from build123d import *

# Parameters (mm, degrees)
F1_DEPTH = 3


with BuildPart() as f1:
    # F0 (on Front) → F1 (new body)
    with BuildSketch(Plane.XZ):
        Polygon((-52.314732, 2.8), (-52.314732, 0), (-52.314732, -2.8), (-55.314732, -2.8), (-55.314732, -12.8), (-52.314732, -12.8), (-52.314732, -19.8), (-35.314732, -19.8), (-35.314732, -22.8), (-25.314732, -22.8), (-25.314732, -19.8), (-16.314732, -19.8), (-16.314732, -13.3), (-17.314732, -13.3), (-17.314732, -11.3), (-16.314732, -11.3), (-16.314732, -7.8), (-14.314732, -7.8), (-14.314732, -11.3), (-13.314732, -11.3), (-13.314732, -13.3), (-14.314732, -13.3), (-14.314732, -19.8), (-5.314732, -19.8), (-5.314732, -22.8), (-0.314732, -22.8), (4.685268, -22.8), (4.685268, -19.8), (13.685268, -19.8), (13.685268, -13.3), (12.685268, -13.3), (12.685268, -11.3), (13.685268, -11.3), (13.685268, -7.8), (15.685268, -7.8), (15.685268, -11.3), (16.685268, -11.3), (16.685268, -13.3), (15.685268, -13.3), (15.685268, -19.8), (24.685268, -19.8), (24.685268, -22.8), (34.685268, -22.8), (34.685268, -19.8), (51.685268, -19.8), (51.685268, -12.8), (54.685268, -12.8), (54.685268, -2.8), (51.685268, -2.8), (51.685268, 0), (51.685268, 2.8), (54.685268, 2.8), (54.685268, 12.8), (51.685268, 12.8), (51.685268, 19.8), (34.685268, 19.8), (34.685268, 22.8), (24.685268, 22.8), (24.685268, 19.8), (15.685268, 19.8), (15.685268, 13.3), (16.685268, 13.3), (16.685268, 11.3), (15.685268, 11.3), (15.685268, 7.8), (13.685268, 7.8), (13.685268, 11.3), (12.685268, 11.3), (12.685268, 13.3), (13.685268, 13.3), (13.685268, 19.8), (4.685268, 19.8), (4.685268, 22.8), (-0.314732, 22.8), (-5.314732, 22.8), (-5.314732, 19.8), (-14.314732, 19.8), (-14.314732, 13.3), (-13.314732, 13.3), (-13.314732, 11.3), (-14.314732, 11.3), (-14.314732, 7.8), (-16.314732, 7.8), (-16.314732, 11.3), (-17.314732, 11.3), (-17.314732, 13.3), (-16.314732, 13.3), (-16.314732, 19.8), (-25.314732, 19.8), (-25.314732, 22.8), (-35.314732, 22.8), (-35.314732, 19.8), (-52.314732, 19.8), (-52.314732, 12.8), (-55.314732, 12.8), (-55.314732, 2.8), align=None)
    extrude(amount=F1_DEPTH)


solid = f1.part
The listing builds one solid part. Answer for the finished solid, in the listing's coordinates (mm). A direction names the side the tool comes from. Coordinates: 2 decimals unless noted, no trailing zeros. Write each loop counter-clockwise with the first axis right and the second up, starting at its lowest first coordinate (ties: lowest second). Pieces come first, ordered by that corner, then holes. Notation, with made-up numbers: (-13, 76.5) - (21, 76.5) arc R11 ccw to (21, 83.5) - close; hole circle Ø3 at (28, 3). An arc over 180 degrees is marked (long way). Answer as CSV lines item,"result".
1. Find section A-A (z = -15.5). Give the vertices of the cut face in (x, y), plus the area to 3 significant figures.
Computed values:
outline,"(-52.31, -3) - (-16.31, -3) - (-16.31, 0) - (-52.31, 0) - close; (-14.31, -3) - (13.69, -3) - (13.69, 0) - (-14.31, 0) - close; (15.69, -3) - (51.69, -3) - (51.69, 0) - (15.69, 0) - close"
area,"300 mm²"
2. Determine the mould class of faces 4 (the flat face through (-44, -1, -19.8)), 5 (the flat face through (16.685, -1, -12)), 6 (the flat face through (15.685, -1, 17)), 7 (the flat face through (51.685, -1, -16)) for opening direction X: +X half, -X half, draft (parallel to the pull), parting line (faces both ways), or undercut.
Computed values:
face 4,"draft"
face 5,"undercut"
face 6,"undercut"
face 7,"+X half"
3. A tool of negligible diameter and unlimited length cuts with its end or side. For faces 1 (the flat face through (-13.315, -1, -12)), 2 (the flat face through (20, -1, 19.8)), 3 (the flat face through (-21, -1, -19.8)), from which of +Z, -Z, +X, -X, +Y, -Y can it reach the whole face along a straight path? Write none if from no direction.
Computed values:
face 1,"+Y, -Y"
face 2,"+Z, +Y, -Y"
face 3,"-Z, +Y, -Y"
4. Given P1, Ø1.1, axis at x = 13.5, y = -1, coming from the +Z side; P2, Ø10, axis at x = 37.5, z = -8.5, coming from the +Y side; P3, Ø1.1, axis at x = -13.5, y = -1, coming from the -Z side; P4, Ø1, axis at y = -2, z = -2, coming from the +X side, each flat-ended and moving along its own axis, determine where each tip first touches the part or whether it passes through.
Computed values:
P1,"stops at z = 19.8"
P2,"stops at y = 0"
P3,"stops at z = -19.8"
P4,"stops at x = 51.69"
5. Find section B-B (x = -23.5). Give the vertices of the cut face in (y, z), plus the area to 3 significant figures.
Computed values:
outline,"(-3, -19.8) - (0, -19.8) - (0, 19.8) - (-3, 19.8) - close"
area,"119 mm²"
6. Straight lines are drawn through the part: line 1 (X direction, y = -0.4, z = 11); line 2 (X direction, y = -1.6, z = 21.5); line 3 (Z direction, x = 7.5, y = -2.5). For each, find the intervals that lie inside material, in ascending order. Write a range as [from, to].
Computed values:
line 1,"x = [-55.31, -16.31], [-14.31, 13.69], [15.69, 54.69]"
line 2,"x = [-35.31, -25.31], [-5.31, 4.69], [24.69, 34.69]"
line 3,"z = [-19.8, 19.8]"
